from build123d import *

# Parameters (mm, degrees)
BOSS_EXTRUDE1_DEPTH     = 125
FILLET1_R               = 1
FILLET2_R               = 2
SKETCH3_R               = 1.6
CUT_EXTRUDE1_DEPTH      = 221.054985344
CUT_EXTRUDE2_DEPTH      = 221.054985344
CUT_EXTRUDE2_DEPTH_BACK = 221.054985344


with BuildPart() as part:
    # Sketch2 → Boss-Extrude1 (new body)
    with BuildSketch(Plane(origin=(0, 0, 0), x_dir=(1, 0, 0), z_dir=(0, 1, 0))):
        Polygon((174.628739257, -52.498316328), (174.628739257, -2.498316328), (162.628739257, -2.498316328), (162.628739257, -4.498316328), (172.628739257, -4.498316328), (172.628739257, -52.498316328), align=None)
    extrude(amount=BOSS_EXTRUDE1_DEPTH)

    # Fillet1
    fillet1_edges = [part.edges().sort_by_distance(p)[0] for p in [
        (172.628739257, 62.5, 52.498316328),
        (162.628739257, 62.5, 4.498316328),
    ]]
    fillet(fillet1_edges, radius=FILLET1_R)

    # Fillet2
    fillet2_edges = [part.edges().sort_by_distance(p)[0] for p in [
        (172.628739257, 62.5, 4.498316328),
    ]]
    fillet(fillet2_edges, radius=FILLET2_R)

    # Sketch3 → Cut-Extrude1 (cut, through all)
    with BuildSketch(Plane.XY.offset(4.498316328)):
        with Locations((167.128739257, 20)):
            Circle(SKETCH3_R)
        with Locations((167.128739257, 105)):
            Circle(SKETCH3_R)
    extrude(amount=-CUT_EXTRUDE1_DEPTH, mode=Mode.SUBTRACT)

    # Sketch4 → Cut-Extrude2 (cut, two sides: drawn at the far end of the back side and taken through both)
    with BuildSketch(Plane.XY.offset(4.498316328).offset(-CUT_EXTRUDE2_DEPTH_BACK)):
        Polygon((174.628739257, 0), (162.628739257, 12), (162.628739257, 0), align=None)
    extrude(amount=CUT_EXTRUDE2_DEPTH + CUT_EXTRUDE2_DEPTH_BACK, mode=Mode.SUBTRACT)


solid = part.part
Build history of the part. All positions in model axes, mm. A direction names the side the tool comes from. Give positions to 0.01 mm unless a question says otherwise; leave off trailing zeros. Write each loop counter-clockwise with the first axis right and the second up, starting at its lowest first coordinate (ties: lowest second). Pieces come first, ordered by that corner, then holes. Notation, with made-up numbers: (7.5, -12) - (11.5, -12) arc R21 ccw to (11.5, 14) - close; hole circle Ø4 at (73, 22.5). An arc over 180 degrees is marked (long way). Use one line per item in the form item = value. Start each with the question number.
1. Band-saw the part on B-B on y = 62. Write the cut outline in (x, z).
2. Two-plate mould, pull along X, no slides. Class faces 3 (the face through (173, 125, 22)), 4 (the face through (172.629, 63, 29)), 5 (the face through (174.629, 62, 28)), 6 (the face through (165.95, 21.08, 3.51)): released by +X, released by -X, zero draft, split by the parting line, or undercut.
3. Band-saw the part on C-C on x = 167.5. Write the cut outline in (y, z).
4. Band-saw the part on D-D on z = 23.5. Write the cut outline in (x, y), plus the area to 3 significant figures.
5. Probe line 1 (X direction, y = 105, z = 3); line 2 (X direction, y = 115, z = 46); line 3 (Z direction, x = 168.75, y = 118.5). List the from-to ranges inside material, lowest first. Write a range as [from, to].
6. Drop flat-ended pins along their axis: pin 1 Ø13.5 at (y, z) = (84, 28.5) entering from -X; pin 2 Ø4 at (x, y) = (167.13, 105) entering from +Z; pin 3 Ø3 at (x, y) = (170, 87.5) entering from +Z. Give the stop position or say it passes through.
7. Band-saw the part on A-A on y = 105. Write the cut outline in (x, z).
8. 3-axis set-ups, long thin cutter, end or side, ignore diameter. For faces 1 (the face through (165.53, 105.07, 3.51)), 2 (the face through (167, 64, 4.498)): which of +Z, -Z, +X, -X, +Y, -Y reach the whole face in a straight line?
Conclusion:
q1.outline = (162.63, 2.5) - (174.63, 2.5) - (174.63, 52.5) - (173.63, 52.5) arc R1 ccw to (172.63, 51.5) - (172.63, 6.5) arc R2 cw to (170.63, 4.5) - (163.63, 4.5) arc R1 ccw to (162.63, 3.5) - close
q2.face_3 = zero draft
q2.face_4 = released by -X
q2.face_5 = released by +X
q2.face_6 = undercut
q3.outline = (7.13, 2.5) - (18.44, 2.5) - (18.44, 4.5) - (7.13, 4.5) - close; (21.56, 2.5) - (103.44, 2.5) - (103.44, 4.5) - (21.56, 4.5) - close; (106.56, 2.5) - (125, 2.5) - (125, 4.5) - (106.56, 4.5) - close
q4.outline = (172.63, 2) - (174.63, 0) - (174.63, 125) - (172.63, 125) - close
q4.area = 248 mm²
q5.line_1 = [162.63, 165.53], [168.73, 174.63]
q5.line_2 = [172.63, 174.63]
q5.line_3 = [2.5, 4.5]
q6.pin_1 = 172.63
q6.pin_2 = 4.5
q6.pin_3 = 4.7
q7.outline = (162.63, 2.5) - (165.53, 2.5) - (165.53, 4.5) - (163.63, 4.5) arc R1 ccw to (162.63, 3.5) - close; (168.73, 2.5) - (174.63, 2.5) - (174.63, 52.5) - (173.63, 52.5) arc R1 ccw to (172.63, 51.5) - (172.63, 6.5) arc R2 cw to (170.63, 4.5) - (168.73, 4.5) - close
q8.face_1 = +Z, -Z
q8.face_2 = +Z, -X, +Y, -Y
